```python
from build123d import *

# Parameters (mm, degrees)
SKETCH1_W                 = 50.8
SKETCH1_H                 = 12.7
BOSS_EXTRUDE1_DEPTH       = 62.738
F_8_32_TAPPED_HOLE1_D     = 3.4544
F_8_32_TAPPED_HOLE1_DEPTH = 17.6276
F_8_32_TAPPED_HOLE1_TIP   = 1.037806461
F_2_56_TAPPED_HOLE1_D     = 1.778
F_2_56_TAPPED_HOLE1_DEPTH = 12.7
F_2_56_TAPPED_HOLE1_TIP   = 0.53416509
F_2_56_TAPPED_HOLE2_D     = 1.778
F_2_56_TAPPED_HOLE2_DEPTH = 10.8204
F_2_56_TAPPED_HOLE2_TIP   = 0.53416509


with BuildPart() as part:
    # Sketch1 → Boss-Extrude1 (new body)
    with BuildSketch(Plane(origin=(0, 0, 0), x_dir=(1, 0, 0), z_dir=(0, 1, 0))):
        with Locations((25.4, -6.35)):
            Rectangle(SKETCH1_W, SKETCH1_H)
    extrude(amount=BOSS_EXTRUDE1_DEPTH)

    # #8-32 Tapped Hole1
    with Locations(Plane(origin=(0, 0, 0), x_dir=(-1, 0, 0), z_dir=(0, -1, 0))):
        with Locations((-6.35, -6.35), (-44.45, -6.35)):
            Hole(F_8_32_TAPPED_HOLE1_D / 2, depth=F_8_32_TAPPED_HOLE1_DEPTH)
            with Locations((0, 0, -(F_8_32_TAPPED_HOLE1_DEPTH + F_8_32_TAPPED_HOLE1_TIP / 2))):  # 118° drill point
                Cone(0, F_8_32_TAPPED_HOLE1_D / 2, F_8_32_TAPPED_HOLE1_TIP, mode=Mode.SUBTRACT)

    # #2-56 Tapped Hole1
    with Locations(Plane(origin=(0, 62.738, 0), x_dir=(1, 0, 0), z_dir=(0, 1, 0))):
        with Locations((7.9375, -6.35), (42.8625, -6.35)):
            Hole(F_2_56_TAPPED_HOLE1_D / 2, depth=F_2_56_TAPPED_HOLE1_DEPTH)
            with Locations((0, 0, -(F_2_56_TAPPED_HOLE1_DEPTH + F_2_56_TAPPED_HOLE1_TIP / 2))):  # 118° drill point
                Cone(0, F_2_56_TAPPED_HOLE1_D / 2, F_2_56_TAPPED_HOLE1_TIP, mode=Mode.SUBTRACT)

    # #2-56 Tapped Hole2
    with Locations(Plane.XY.offset(12.7)):
        with Locations((30.48, 59.436), (45.72, 59.436)):
            Hole(F_2_56_TAPPED_HOLE2_D / 2, depth=F_2_56_TAPPED_HOLE2_DEPTH)
            with Locations((0, 0, -(F_2_56_TAPPED_HOLE2_DEPTH + F_2_56_TAPPED_HOLE2_TIP / 2))):  # 118° drill point
                Cone(0, F_2_56_TAPPED_HOLE2_D / 2, F_2_56_TAPPED_HOLE2_TIP, mode=Mode.SUBTRACT)


solid = part.part
```
Input: part model. Units: mm. Frame: model coordinates. A direction names the side the tool comes from. Round coordinates to 2 decimals unless told otherwise and drop trailing zeros. Write each loop counter-clockwise with the first axis right and the second up, starting at its lowest first coordinate (ties: lowest second). Pieces come first, ordered by that corner, then holes. Notation, with made-up numbers: (50.25, 72.25) - (56.25, 72.25) arc R17 ccw to (56.25, 102.25) - close; hole circle Ø10 at (24.5, 35). An arc over 180 degrees is marked (long way). Write item = value, one per line.
(1) Section query A-A on y = 9. Output: boundary loops of the cut face in (x, z).
Geometry check:
outline = (0, 0) - (50.8, 0) - (50.8, 12.7) - (0, 12.7) - close; hole circle Ø3.45 at (6.35, 6.35); hole circle Ø3.45 at (44.45, 6.35)
(2) Material intervals for probe 1 along X at (y, z) = (5.5, 6.35); probe 2 along X at (y, z) = (55.75, 6.35); probe 3 along Y at (x, z) = (30.48, 6) (3 decimals), sorted ascending.
Geometry check:
probe_1 = 0 to 4.62, 8.08 to 42.72, 46.18 to 50.8
probe_2 = 0 to 7.05, 8.83 to 41.97, 43.75 to 50.8
probe_3 = 0 to 58.547, 60.325 to 62.738
(3) Access query for faces 1 (the cylindrical face through (8.643, 56.299, 6.891)), 2 (the cylindrical face through (31.135, 60.037, 7.214)), 3 (the cylindrical face through (43.18, 8.94, 5.18)). Directions: +Z, -Z, +X, -X, +Y, -Y. A direction counts if a zero-diameter tool reaches every point of the face in a straight line with its end or side. Return the directions, or none.
Geometry check:
face_1 = +Y
face_2 = +Z
face_3 = -Y
(4) Contact query for flat-ended pins moving along their axis: pin 1 Ø1.4 at (x, y) = (45.72, 59.436) entering from +Z; pin 2 Ø1.1 at (x, z) = (42.86, 6.35) entering from +Y. Output: stop coordinate, or through.
Geometry check:
pin_1 = 1.77
pin_2 = 49.84
(5) Pull-direction query (Z, two-part tool) for faces 4 (the flat face through (25, 31, 0)), 5 (the flat face through (25, 31, 12.7)), 6 (the cylindrical face through (6.125, 8.937, 4.637)), 7 (the cylindrical face through (45.836, 60.317, 7.214)); classes: +Z half, -Z half, draft (parallel to the pull), parting line (faces both ways), or undercut.
Geometry check:
face_4 = -Z half
face_5 = +Z half
face_6 = undercut
face_7 = draft
